```python
from build123d import *

# Parameters (mm, degrees)
SKETCH_1_R          = 1.5
EXTRUDE_1_DEPTH     = 2
SKETCH_3_R          = 0.5
CUT_EXTRUDE_3_DEPTH = 10
FILLET_1_R          = 1


with BuildPart() as part:
    # 草图1 → 凸台-拉伸1 (new body)
    with BuildSketch(Plane.XY):
        Polygon((5, 45), (-5, 45), (-5, 15), (-5, 7.1), (5.1, 7.1), (5.1, -5), (15, -5), (35, -5), (35, 5), align=None)
        with Locations((0, 20)):
            Circle(SKETCH_1_R, mode=Mode.SUBTRACT)
        with Locations((15, 0)):
            Circle(SKETCH_1_R, mode=Mode.SUBTRACT)
        with Locations((30, 0)):
            Circle(SKETCH_1_R, mode=Mode.SUBTRACT)
        with Locations((0, 35)):
            Circle(SKETCH_1_R, mode=Mode.SUBTRACT)
    extrude(amount=EXTRUDE_1_DEPTH)

    # 草图3 → 切除-拉伸3 (cut)
    with BuildSketch(Plane.XY.offset(2)):
        with Locations((5.1, 7.1)):
            Circle(SKETCH_3_R)
    extrude(amount=-CUT_EXTRUDE_3_DEPTH, mode=Mode.SUBTRACT)

    # 圆角1
    fillet_1_edges = [part.edges().sort_by_distance(p)[0] for p in [
        (-5, 45, 1),
        (5, 45, 1),
        (35, 5, 1),
        (35, -5, 1),
        (5.1, -5, 1),
        (-5, 7.1, 1),
    ]]
    fillet(fillet_1_edges, radius=FILLET_1_R)


solid = part.part
```
Source: CAD feature listing. Evaluate the final solid. Frame: model axes, mm. A direction names the side the tool comes from. Round coordinates to 2 decimals unless told otherwise and drop trailing zeros. Loops run counter-clockwise (first coordinate to the right, second up) from the corner with the lowest first, then second, coordinate; pieces in that order, holes last. Notation, with made-up numbers: M 63,27.25 L 118,27.25 A20 cw 118,35.25 Z; hole C 22.25,72 d2. An arc over 180 degrees is marked long. Use a Markdown table: item, result. Add a question column.
1. Section query A-A on y = 35. Return the cut outline in (x, z), then the cut area to 3 significant figures.
2. Section query B-B on x = 30. Return the cut outline in (y, z), then the cut area to 3 significant figures.
3. Line query: line 1 (Y direction, x = 0, z = 0.75); line 2 (X direction, y = 36, z = 1.8); line 3 (X direction, y = -3, z = 0.65). Output: solid intervals per line, ascending.
4. Section query D-D on y = 0. Return the cut outline in (x, z).
5. Section query C-C on z = 1.35. Return the cut outline in (x, y).
6. Reachability of faces 4 (the flat face through (10, 15, 0)), 5 (the flat face through (0, 7.1, 1)) from +Z, -Z, +X, -X, +Y, -Y: full face, straight path, thin tool, end or side. Return the list, or none.
7. Contact query for flat-ended pins moving along their axis: P1, Ø1, axis at y = 0.5, z = 1, coming from the -X side; P2, Ø1, axis at x = 2, z = 1, coming from the -Y side. Output: stop coordinate, or through.
8. Mould query, pull axis Y, two halves, no side actions, for faces 1 (the flat face through (-5, 26, 1)), 2 (the flat face through (0, 45, 1)), 3 (the cylindrical face through (5.5, 7.4, 1)). Classes: pulls with the +Y half, pulls with the -Y half, needs draft (parallel to the pull), parting line crosses it, or undercut.
Reported:
| question | item | result |
|---|---|---|
| 1 | outline | M -5,0 L -1.5,0 L -1.5,2 L -5,2 Z; M 1.5,0 L 12.5,0 L 12.5,2 L 1.5,2 Z |
| 1 | area | 29.0 mm² |
| 2 | outline | M -5,0 L -1.5,0 L -1.5,2 L -5,2 Z; M 1.5,0 L 11.67,0 L 11.67,2 L 1.5,2 Z |
| 2 | area | 27.3 mm² |
| 3 | line 1 | y = 7.1 to 18.5, 21.5 to 33.5, 36.5 to 45 |
| 3 | line 2 | x = -5 to -1.12, 1.12 to 11.75 |
| 3 | line 3 | x = 5.1 to 35 |
| 4 | outline | M 5.1,0 L 13.5,0 L 13.5,2 L 5.1,2 Z; M 16.5,0 L 28.5,0 L 28.5,2 L 16.5,2 Z; M 31.5,0 L 35,0 L 35,2 L 31.5,2 Z |
| 5 | outline | M -5,8.1 A1 ccw -4,7.1 L 4.6,7.1 A0.5 cw long 5.1,6.6 L 5.1,-4 A1 ccw 6.1,-5 L 34,-5 A1 ccw 35,-4 L 35,4.67 A1 ccw 34.8,5.27 L 5.3,44.6 A1 ccw 4.5,45 L -4,45 A1 ccw -5,44 Z; hole C 0,20 d3; hole C 0,35 d3; hole C 15,0 d3; hole C 30,0 d3 |
| 6 | face 4 | -Z, +X, -X, +Y, -Y |
| 6 | face 5 | +Z, -Z, -X, -Y |
| 7 | P1 | stops at x = 5.1 |
| 7 | P2 | stops at y = 7.1 |
| 8 | face 1 | needs draft |
| 8 | face 2 | pulls with the +Y half |
| 8 | face 3 | undercut |
